from build123d import *

# Parameters (mm, degrees)
F0_W     = 34
F0_H     = 74
F1_DEPTH = 25
F2_T     = -2
F3_R     = 1
F4_DEPTH = 25
F5_R     = 1
F6_DEPTH = 5
F8_DEPTH = 25


with BuildPart() as f1:
    # F0 (on Top) → F1 (new body)
    with BuildSketch(Plane.XY):
        Rectangle(F0_W, F0_H)
    extrude(amount=F1_DEPTH)

    # F2
    f2_openings = [f1.faces().sort_by_distance(p)[0] for p in [
        (0, 0, 25),
    ]]
    offset(amount=F2_T, openings=f2_openings)

    # F3 (on face) → F4 (cut)
    with BuildSketch(Plane.XY.offset(2)):
        with Locations((13, 33)):
            Circle(F3_R)
        with Locations((-13, 33)):
            Circle(F3_R)
        with Locations((13, -33)):
            Circle(F3_R)
        with Locations((-13, -33)):
            Circle(F3_R)
    extrude(amount=-F4_DEPTH, mode=Mode.SUBTRACT)

    # F5 (on face) → F6 (join)
    with BuildSketch(Plane.XY.offset(2)):
        with BuildLine():
            Line((15, -35), (15, -30))
            ThreePointArc((15, -30), (11.4644660941, -31.4644660941), (10, -35))
            Line((10, -35), (15, -35))
        make_face()
        with Locations((13, -33)):
            Circle(F5_R, mode=Mode.SUBTRACT)
        with BuildLine():
            ThreePointArc((-10, -35), (-11.4644660941, -31.4644660941), (-15, -30))
            Line((-15, -30), (-15, -35))
            Line((-15, -35), (-10, -35))
        make_face()
        with Locations((-13, -33)):
            Circle(F5_R, mode=Mode.SUBTRACT)
        with BuildLine():
            ThreePointArc((-15, 30), (-11.4644660941, 31.4644660941), (-10, 35))
            Line((-10, 35), (-15, 35))
            Line((-15, 35), (-15, 30))
        make_face()
        with Locations((-13, 33)):
            Circle(F5_R, mode=Mode.SUBTRACT)
        with BuildLine():
            Line((15, 35), (10, 35))
            ThreePointArc((10, 35), (11.4644660941, 31.4644660941), (15, 30))
            Line((15, 30), (15, 35))
        make_face()
        with Locations((13, 33)):
            Circle(F5_R, mode=Mode.SUBTRACT)
    extrude(amount=F6_DEPTH)

    # F7 (on face) → F8 (cut)
    with BuildSketch(Plane(origin=(0, 0, 0), x_dir=(1, 0, 0), z_dir=(0, 0, -1))):
        Polygon((4, 22), (4, 30), (-4, 30), (-4, 22), (-12, 22), (-12, 12), (-4, 12), (-4, 4), (4, 4), (4, 12), (12, 12), (12, 22), align=None)
    extrude(amount=-F8_DEPTH, mode=Mode.SUBTRACT)


solid = f1.part
Geometry check sheet. Reference: the model listing, model coordinates, mm. A direction names the side the tool comes from. Coordinates: 2 decimals unless noted, no trailing zeros. Write each loop counter-clockwise with the first axis right and the second up, starting at its lowest first coordinate (ties: lowest second). Pieces come first, ordered by that corner, then holes. Notation, with made-up numbers: (49, 20) -> (59, 20) arc R22 cw to (59, 30) -> close; hole circle Ø6 at (27.25, 9). An arc over 180 degrees is marked (long way). One line per question, with ' | ' between items.
1. Cross-section at A-A on x = -6. Record the cut outline in (y, z).
Answers:
outline: (-37, 0) -> (-22, 0) -> (-22, 2) -> (-35, 2) -> (-35, 25) -> (-37, 25) -> close; (-12, 0) -> (37, 0) -> (37, 25) -> (35, 25) -> (35, 2) -> (-12, 2) -> close
2. Thickness scan on probe 1 along Y at (x, z) = (13, 1.2); probe 2 along Y at (x, z) = (2, 2.5); probe 3 along X at (y, z) = (-10, 23.75). Record the ranges inside material, lowest first. Write a range as from..to.
Answers:
probe 1: y = -37..-34, -32..32, 34..37 | probe 2: y = -37..-35, 35..37 | probe 3: x = -17..-15, 15..17
3. Depth check by flat-ended pin: pin 1 Ø10 at (x, y) = (-5, -7) entering from +Z; pin 2 Ø1.5 at (x, y) = (13.5, -33.5) entering from +Z. Enter the tip coordinate at first touch or a pass-through.
Answers:
pin 1: stops at z = 2 | pin 2: stops at z = 7
4. Set-up check for faces 3 (the flat face through (12, -32, 7)), 4 (the flat face through (0, -30, 1)), 5 (the flat face through (17, -1, 12)): record each of +Z, -Z, +X, -X, +Y, -Y from which the full face is reachable in a straight line by a thin tool's end or side.
Answers:
face 3: +Z | face 4: +Z, -Z | face 5: +Z, -Z, +X, +Y, -Y
5. Cross-section at B-B on y = -18. Record the cut outline in (x, z), and give its area (3 significant figures).
Answers:
outline: (-17, 0) -> (-12, 0) -> (-12, 2) -> (-15, 2) -> (-15, 25) -> (-17, 25) -> close; (12, 0) -> (17, 0) -> (17, 25) -> (15, 25) -> (15, 2) -> (12, 2) -> close | area: 112 mm²
6. Draft check along Y on faces 1 (the flat face through (-15, 0, 13)), 2 (the flat face through (-15.2, 2.9, 25)). Enter one of: +Y half, -Y half, draft (parallel to the pull), parting line (faces both ways), or undercut.
Answers:
face 1: undercut | face 2: draft
7. Cross-section at D-D on z = 5.75. Record the cut outline in (x, y), and give its area (3 significant figures).
Answers:
outline: (-17, -37) -> (17, -37) -> (17, 37) -> (-17, 37) -> close; hole (-15, -30) arc R5 cw to (-10, -35) -> (10, -35) arc R5 cw to (15, -30) -> (15, 30) arc R5 cw to (10, 35) -> (-10, 35) arc R5 cw to (-15, 30) -> close; hole circle Ø2 at (-13, -33); hole circle Ø2 at (-13, 33); hole circle Ø2 at (13, -33); hole circle Ø2 at (13, 33) | area: 482 mm²
8. Cross-section at C-C on z = 12. Record the cut outline in (x, y), and give its area (3 significant figures).
Answers:
outline: (-17, -37) -> (17, -37) -> (17, 37) -> (-17, 37) -> close; hole (-15, -35) -> (15, -35) -> (15, 35) -> (-15, 35) -> close | area: 416 mm²
